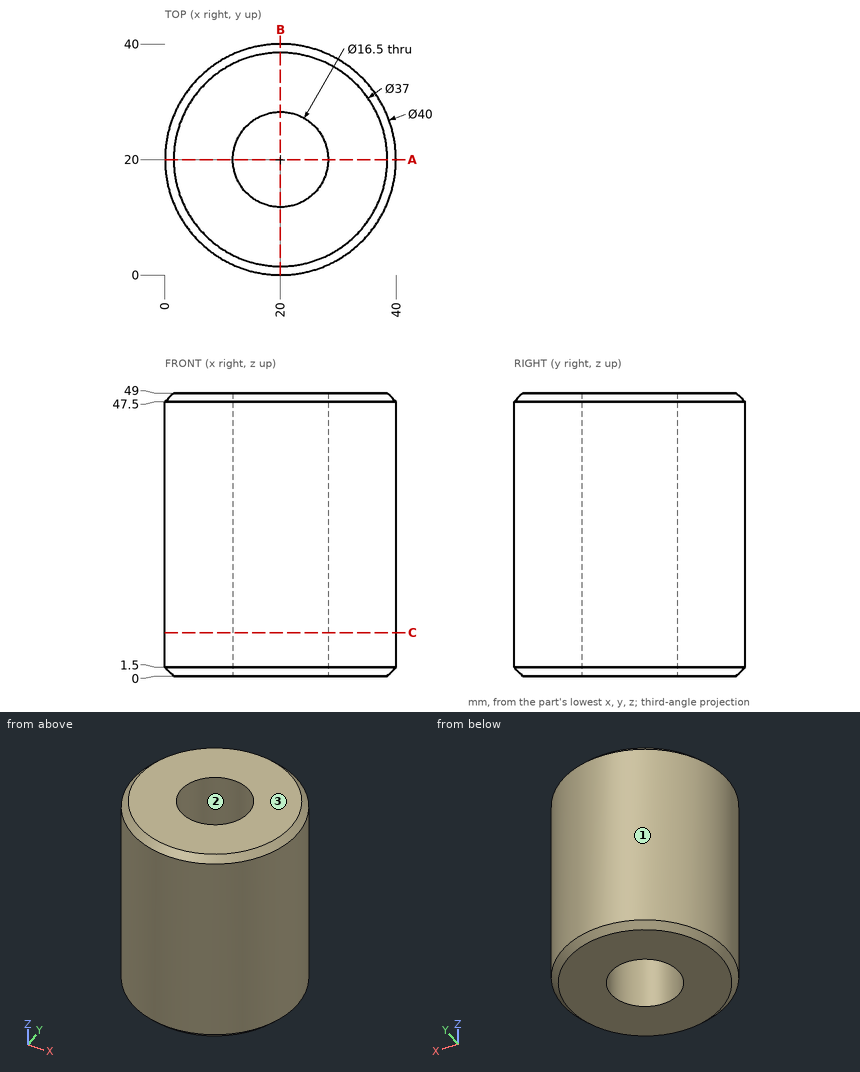
The figure shows three views and two pictorial views of one solid part (mm, origin at its lowest corner). Answer the questions. Coordinates: 2 decimals unless noted, no trailing zeros. Write each loop counter-clockwise with the first axis right and the second up, starting at its lowest first coordinate (ties: lowest second). Pieces come first, ordered by that corner, then holes. Notation, with made-up numbers: (72, 74.25) -> (109, 74.25) arc R20 ccw to (109, 87.25) -> close; hole circle Ø3 at (78, 24). An arc over 180 degrees is marked (long way). Return JSON: item names as keys, results as strings.
(1) Each of these flat-tipped pins is pushed along its axis until it touches: P1, Ø6, axis at y = 6.5, z = 17, coming from the +X side; P2, Ø4, axis at x = 32, z = 31, coming from the +Y side; P3, Ø10, axis at x = 16, z = 21.5, coming from the +Y side. Where does it stop, or does it pass through?
Answers below:
{"P1": "x = 37.02", "P2": "y = 37.32", "P3": "y = 40"}
(2) The part is cut by section A-A on y = 20. Give the vertices of the cut face in (x, z), then the cut area to 3 significant figures.
Answers below:
{"outline": "(0, 1.5) -> (1.5, 0) -> (11.75, 0) -> (11.75, 49) -> (1.5, 49) -> (0, 47.5) -> close; (28.25, 0) -> (38.5, 0) -> (40, 1.5) -> (40, 47.5) -> (38.5, 49) -> (28.25, 49) -> close", "area": "1,150 mm^2"}
(3) For a pull along Y with two mould halves and no side action, classify the marked faces 1, 2 and 3 as pulls with the +Y half, pulls with the -Y half, needs draft (parallel to the pull), parting line crosses it, or undercut.
Answers below:
{"face 1": "parting line crosses it", "face 2": "undercut", "face 3": "needs draft"}
(4) Consider line 1 along Y through (x, z) = (20, 19); line 2 along X through (y, z) = (27, 12) (3 decimals); line 3 along X through (y, z) = (15.5, 3). Determine where each line is inside the solid, lowest interval first. Write a range as from..to.
Answers below:
{"line 1": "0..11.75, 28.25..40", "line 2": "1.265..15.634, 24.366..38.735", "line 3": "0.51..13.09, 26.91..39.49"}
(5) The part is cut by section C-C on z = 7.5. Give the vertices of the cut face in (x, y).
Answers below:
{"outline": "circle Ø40 at (20, 20); hole circle Ø16.5 at (20, 20)"}
